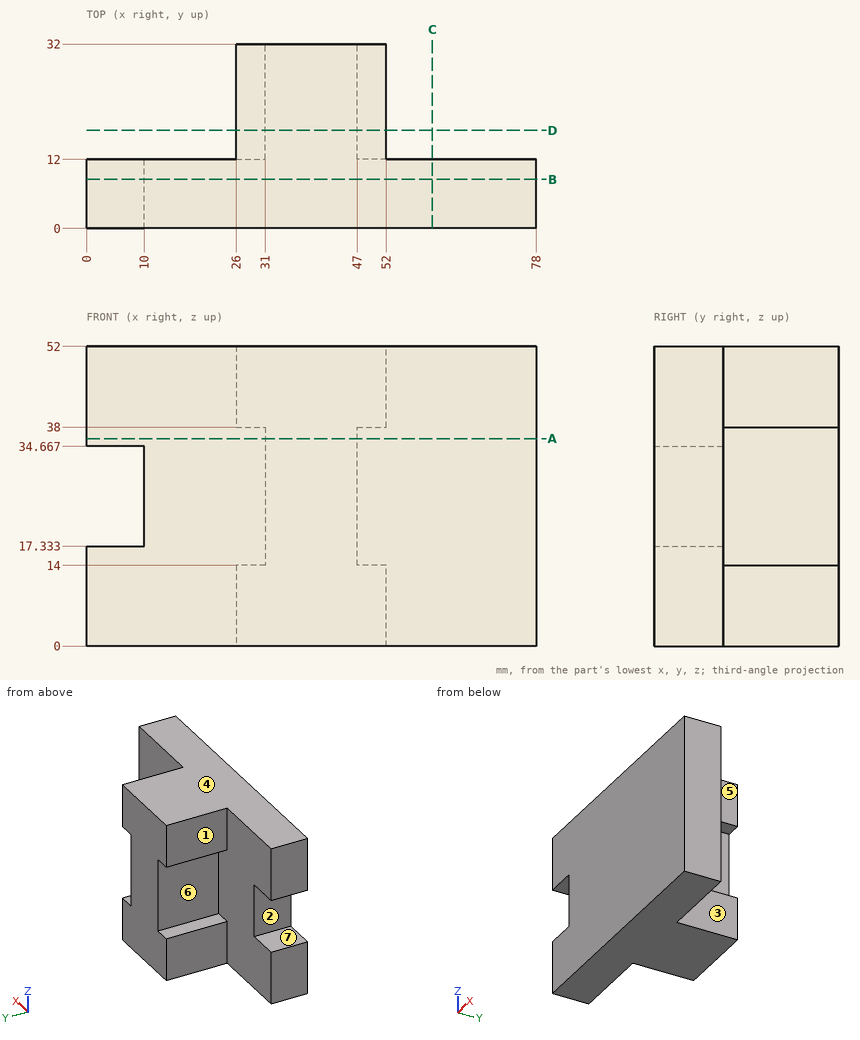
The figure shows three views and two pictorial views of one solid part (mm, origin at its lowest corner). Answer the questions. A direction names the side the tool comes from. Coordinates: 2 decimals unless noted, no trailing zeros. Write each loop counter-clockwise with the first axis right and the second up, starting at its lowest first coordinate (ties: lowest second). Pieces come first, ordered by that corner, then holes.
1. The part is cut by section D-D, the plane y = 17. Write down the section's boundary in (x, z).
Results list:
outline: (26, 0) - (52, 0) - (52, 14) - (47, 14) - (47, 38) - (52, 38) - (52, 52) - (26, 52) - (26, 38) - (31, 38) - (31, 14) - (26, 14) - close
2. The part is cut by section B-B, the plane y = 8.5. Write down the section's boundary in (x, z).
Results list:
outline: (0, 0) - (78, 0) - (78, 52) - (0, 52) - (0, 34.67) - (10, 34.67) - (10, 17.33) - (0, 17.33) - close
3. Consider line 1 along X through (y, z) = (13.5, 24.5); line 2 along Y through (x, z) = (3, 12.5); line 3 along X through (y, z) = (9, 19.5). Determine where each line is inside the solid, lowest interval first.
Results list:
line 1: x = 31 to 47
line 2: y = 0 to 12
line 3: x = 10 to 78
4. The part is cut by section C-C, the plane x = 60. Write down the section's boundary in (y, z), and give its area (3 significant figures).
Results list:
outline: (0, 0) - (12, 0) - (12, 52) - (0, 52) - close
area: 624 mm2
5. For a pull along Z with two mould halves and no side action, classify the marked faces 4, 5, 6 and 7 as +Z half, -Z half, draft (parallel to the pull), parting line (faces both ways), or undercut.
Results list:
face 4: +Z half
face 5: draft
face 6: undercut
face 7: undercut
6. Flat-ended cylindrical pins translate along their axes: pin 1 (10 mm diameter, centred on x = 16, z = 10.5, fed in from -Y); pin 2 (4 mm diameter, centred on y = 26.5, z = 7, fed in from +X); pin 3 (11 mm diameter, centred on y = 24, z = 4, fed in from -X); pin 4 (3 mm diameter, centred on y = 25, z = 16.5, fed in from -X). Find the tip coordinate at first contact, or state that the pin passes through.
Results list:
pin 1: stops at y = 0
pin 2: stops at x = 52
pin 3: stops at x = 26
pin 4: stops at x = 31
7. The part is cut by section A-A, the plane z = 36. Write down the section's boundary in (x, y).
Results list:
outline: (0, 0) - (78, 0) - (78, 12) - (47, 12) - (47, 32) - (31, 32) - (31, 12) - (0, 12) - close
8. For the marked faces 1, 2 and 3, determine the directions among +Z, -Z, +X, -X, +Y, -Y from which every point of the face is accessible in a straight line to the end or side of a thin tool.
Results list:
face 1: +Z, -Z, -X, +Y
face 2: -X, +Y, -Y
face 3: +Z, -Z, +X, +Y
